from build123d import *

# Parameters (mm, degrees)
SKETCH1_W           = 2.032
SKETCH1_H           = 34.925
BOSS_EXTRUDE1_DEPTH = 609.6
CUT_EXTRUDE1_REACH  = 612.603
SKETCH2_R           = 4.7625
LPATTERN1_COUNT     = 64
LPATTERN1_PITCH     = 19.05


with BuildPart() as part:
    # Sketch1 → Boss-Extrude1 (new, symmetric)
    with BuildSketch(Plane.XY):
        with Locations((1.016, 17.4625)):
            Rectangle(SKETCH1_W, SKETCH1_H)
    extrude(amount=BOSS_EXTRUDE1_DEPTH, both=True)

    # Sketch2 → Cut-Extrude1 (cut, up to next)
    with BuildSketch(Plane.ZY, mode=Mode.PRIVATE) as cut_extrude1_sk1:
        with Locations((600.075, 17.4625)):
            Circle(SKETCH2_R)
    cut_extrude1_tool1 = extrude(cut_extrude1_sk1.sketch, amount=-CUT_EXTRUDE1_REACH, mode=Mode.PRIVATE) & part.part
    cut_extrude1 = cut_extrude1_tool1.solids().sort_by_distance((0, 17.4625, 600.075))[0]
    add(cut_extrude1, mode=Mode.SUBTRACT)

    # LPattern1: Cut-Extrude1 ×64
    with Locations(*[(0, 0, -i * LPATTERN1_PITCH) for i in range(1, LPATTERN1_COUNT)]):
        add(cut_extrude1, mode=Mode.SUBTRACT)


solid = part.part
Geometry check sheet. Reference: the model listing, model coordinates, mm. Round coordinates to 2 decimals unless told otherwise and drop trailing zeros. Answer as a JSON object with one key per item and string values. Group by question number.
Item 1: Thickness scan on line 1 along Y through (x, z) = (0.5, 315) (3 decimals); line 2 along Y through (x, z) = (1.2, -451.5) (3 decimals). Record the ranges inside material, lowest first.
Item 2: Cross-section at A-A, the plane x = 0.45. Count the separate pieces of the cut face and the enclosed holes in it, plus the area to 3 significant figures.
Item 3: Depth check by flat-ended pin: pin 1 Ø8.5 at (y, z) = (17.46, 371.48) entering from +X (3 decimals). Enter the tip coordinate at first touch or a pass-through.
Determined:
{
 "1": {"line 1": "y = 0 to 12.748, 22.177 to 34.925", "line 2": "y = 0 to 14.625, 20.3 to 34.925"},
 "2": {"separate pieces": "1", "enclosed holes": "64", "area": "38,000 mm²"},
 "3": {"pin 1": "passes through"}
}
